Check sheet for the modelled part. Datum: model origin and axes. Units: mm. A direction names the side the tool comes from. Round coordinates to 2 decimals unless told otherwise and drop trailing zeros. Loops run counter-clockwise (first coordinate to the right, second up) from the corner with the lowest first, then second, coordinate; pieces in that order, holes last. Notation, with made-up numbers: (-9.5, 17) -> (2.5, 17) arc R16 ccw to (2.5, 42) -> close; hole circle Ø6 at (40, 44). An arc over 180 degrees is marked (long way). Return JSON: item names as keys, results as strings.
from build123d import *

# Parameters (mm, degrees)
SKETCH_W        = 38
SKETCH_H        = 20
SKETCH_R        = 2.1
PAD_DEPTH       = 22
SKETCH001_R     = 11.2
POCKET_DEPTH    = 8
SKETCH002_R     = 5.1
SKETCH002_R_2   = 1.75
POCKET001_DEPTH = 20
POCKET002_DEPTH = 3.4
FILLET_R        = 2
FILLET001_R     = 0.4


with BuildPart() as part:
    # Sketch → Pad (new body)
    with BuildSketch(Plane.XY):
        with Locations((19, 10)):
            Rectangle(SKETCH_W, SKETCH_H)
        with Locations((4, 15)):
            Circle(SKETCH_R, mode=Mode.SUBTRACT)
        with Locations((4, 5)):
            Circle(SKETCH_R, mode=Mode.SUBTRACT)
        with Locations((34, 15)):
            Circle(SKETCH_R, mode=Mode.SUBTRACT)
        with Locations((34, 5)):
            Circle(SKETCH_R, mode=Mode.SUBTRACT)
    extrude(amount=PAD_DEPTH)

    # Sketch001 (on Face3 of Pad) → Pocket (cut)
    with BuildSketch(Plane.XZ):
        with Locations((19, 11)):
            Circle(SKETCH001_R)
    extrude(amount=-POCKET_DEPTH, mode=Mode.SUBTRACT)

    # Sketch002 (on Face1 of Pocket) → Pocket001 (cut)
    with BuildSketch(Plane(origin=(0, 20, 0), x_dir=(-1, 0, 0), z_dir=(0, 1, 0))):
        with Locations((-19, 11)):
            Circle(SKETCH002_R)
        with Locations((-13.378501, 16.621499)):
            Circle(SKETCH002_R_2)
        with Locations((-24.621499, 5.378501)):
            Circle(SKETCH002_R_2)
        with Locations((-24.621499, 16.621499)):
            Circle(SKETCH002_R_2)
        with Locations((-13.378501, 5.378501)):
            Circle(SKETCH002_R_2)
    extrude(amount=-POCKET001_DEPTH, mode=Mode.SUBTRACT)

    # Sketch003 (on Face4 of Pocket001) → Pocket002 (cut)
    with BuildSketch(Plane.XY.offset(22)):
        Polygon((4, 10.900813), (7.55, 12.950407), (7.55, 17.049593), (4, 19.099187), (0.45, 17.049593), (0.45, 12.950407), align=None)
        Polygon((34, 10.900813), (37.55, 12.950407), (37.55, 17.049593), (34, 19.099187), (30.45, 17.049593), (30.45, 12.950407), align=None)
        Polygon((34, 9.099187), (30.45, 7.049593), (30.45, 2.950407), (34, 0.900813), (37.55, 2.950407), (37.55, 7.049593), align=None)
        Polygon((4, 9.099187), (0.45, 7.049593), (0.45, 2.950407), (4, 0.900813), (7.55, 2.950407), (7.55, 7.049593), align=None)
    extrude(amount=-POCKET002_DEPTH, mode=Mode.SUBTRACT)

    # Fillet
    fillet_edges = [part.edges().sort_by_distance(p)[0] for p in [
        (16.892869, 4, 22),
        (21.107131, 4, 22),
        (21.107131, 4, 0),
        (16.892869, 4, 0),
    ]]
    fillet(fillet_edges, radius=FILLET_R)

    # Fillet001
    fillet001_edges = [part.edges().sort_by_distance(p)[0] for p in [
        (19, 8, 22),
        (13.118392, 8, 22),
        (24.881608, 8, 22),
        (0, 0, 11),
        (33.328043, 0, 0),
        (4.671957, 0, 0),
        (4.671957, 0, 22),
        (33.328043, 0, 22),
        (26.822064, 0, 20.797724),
        (29.421182, 0, 15.10353),
        (29.421182, 0, 6.89647),
        (26.822064, 0, 1.202276),
        (11.177936, 0, 1.202276),
        (7.8, 0, 11),
        (11.177936, 0, 20.797724),
        (38, 0, 11),
        (38, 10, 22),
        (38, 20, 11),
        (38, 10, 0),
        (0, 10, 22),
        (19, 20, 22),
        (0, 20, 11),
        (19, 20, 0),
        (0, 10, 0),
        (13.118392, 8, 0),
        (19, 8, 0),
        (24.881608, 8, 0),
    ]]
    fillet(fillet001_edges, radius=FILLET001_R)


solid = part.part
Q1. Section check D-D (x = 3.5). Record the boundary of the cut face in (y, z), then the cut area to 3 significant figures.
Results list:
{"outline": "(0, 0.4) arc R0.4 ccw to (0.4, 0) -> (2.96, 0) -> (2.96, 18.6) -> (1.19, 18.6) -> (1.19, 22) -> (0.4, 22) arc R0.4 ccw to (0, 21.6) -> close; (7.04, 0) -> (12.96, 0) -> (12.96, 18.6) -> (11.19, 18.6) -> (11.19, 22) -> (8.81, 22) -> (8.81, 18.6) -> (7.04, 18.6) -> close; (17.04, 0) -> (19.6, 0) arc R0.4 ccw to (20, 0.4) -> (20, 21.6) arc R0.4 ccw to (19.6, 22) -> (18.81, 22) -> (18.81, 18.6) -> (17.04, 18.6) -> close", "area": "236 mm^2"}
Q2. Section check B-B (y = 5). Count the separate pieces of the cut face and the enclosed holes in it, then the cut area to 3 significant figures.
Results list:
{"separate pieces": "4", "enclosed holes": "0", "area": "211 mm^2"}
Q3. Section check A-A (x = 19). Record the boundary of the cut face in (y, z), then the cut area to 3 significant figures.
Results list:
{"outline": "(8, 0.4) arc R0.4 ccw to (8.4, 0) -> (19.6, 0) arc R0.4 ccw to (20, 0.4) -> (20, 5.9) -> (8, 5.9) -> close; (8, 16.1) -> (20, 16.1) -> (20, 21.6) arc R0.4 ccw to (19.6, 22) -> (8.4, 22) arc R0.4 ccw to (8, 21.6) -> close", "area": "141 mm^2"}
Q4. Tool access check on faces 1 (the cylindrical face through (31.9, 15.09, 9.17)), 2 (the flat face through (5.75, 1.91, 20.32)), 3 (the flat face through (21, 8, 16)). Record the directions out of +Z, -Z, +X, -X, +Y, -Y that give a thin tool (end or side, any length) a straight path to the whole face; none if there is none.
Results list:
{"face 1": "+Z, -Z", "face 2": "+Z", "face 3": "-Y"}
Q5. Go/stop test with flat-tipped pins: pin 1 (4 mm diameter, centred on x = 13.38, z = 5.38, fed in from +Y); pin 2 (3.5 mm diameter, centred on x = 32.5, y = 6, fed in from +Z); pin 3 (4.5 mm diameter, centred on x = 24.62, z = 5.38, fed in from -Y). Record where each tip stops, or that it passes through.
Results list:
{"pin 1": "y = 20", "pin 2": "z = 18.6", "pin 3": "y = 8"}
Q6. Section check C-C (z = 2). Record the boundary of the cut face in (x, y), then the cut area to 3 significant figures.
Results list:
{"outline": "(0, 0.4) arc R0.4 ccw to (0.4, 0) -> (10.94, 0) arc R0.4 ccw to (11.34, 0.4) -> (11.34, 8) -> (26.66, 8) -> (26.66, 0.4) arc R0.4 ccw to (27.06, 0) -> (37.6, 0) arc R0.4 ccw to (38, 0.4) -> (38, 19.6) arc R0.4 ccw to (37.6, 20) -> (0.4, 20) arc R0.4 ccw to (0, 19.6) -> close; hole circle Ø4.2 at (4, 5); hole circle Ø4.2 at (4, 15); hole circle Ø4.2 at (34, 5); hole circle Ø4.2 at (34, 15)", "area": "582 mm^2"}
Q7. Draft check along X on faces 4 (the cylindrical face through (5.13, 6.77, 9.17)), 5 (the flat face through (33, 0, 11)), 6 (the flat face through (0, 10, 11)), 7 (the flat face through (32, 13, 18.6)). Enter one of: released by +X, released by -X, zero draft, split by the parting line, or undercut.
Results list:
{"face 4": "undercut", "face 5": "zero draft", "face 6": "released by -X", "face 7": "undercut"}
Q8. Material ranges on line 1 (Y direction, x = 34, z = 9.75); line 2 (X direction, y = 16.5, z = 18.75); line 3 (Z direction, x = 19, y = 13.25), recorded low to high.
Results list:
{"line 1": "0 to 2.9, 7.1 to 12.9, 17.1 to 20", "line 2": "0 to 0.45, 7.55 to 30.45, 37.55 to 38", "line 3": "0 to 5.9, 16.1 to 22"}
